The drawing under review shows one solid part. Ordinate dimensions are in mm from its lowest x, y, z. A direction names the side the tool comes from. Give positions to 0.01 mm unless a question says otherwise; leave off trailing zeros. Order: outer loops, then holes, each group sorted by start corner. A loop starts at its lowest first (then second) coordinate and runs counter-clockwise, first axis right, second up. Notation, with made-up numbers: (83.5, 15) -> (93.5, 15) arc R23 ccw to (93.5, 54) -> close; hole circle Ø9 at (75, 24.25). An arc over 180 degrees is marked (long way). One line per item, written item: value. Start each with the question number.
1) Consider section A-A (y = 16.5). State the section outline as (x, z) points.
2) Consider section D-D (y = 20). State the section outline as (x, z) points.
3) Consider section B-B (z = 8.25). State the section outline as (x, y) points.
4) Consider section C-C (x = 5). State the section outline as (y, z) points, plus the area to 3 significant figures.
5) Wall thickness on line 1 along Z through (x, y) = (7.75, 22.75); line 2 along Y through (x, z) = (5, 2.05); line 3 along X through (y, z) = (20, 3.9): over which ranges is each line inside the solid? List them lowest first. Write a range as from..to.
6) For pin 1 (0.9 mm diameter, centred on x = 5, z = 3.5, fed in from -Y); pin 2 (0.9 mm diameter, centred on x = 9, z = 8, fed in from +Y), all flat-tipped, find the tip position at first contact; note any pin that passes through.
7) Tool access review of the marked faces 1, 2 and 3: name each direction out of +Z, -Z, +X, -X, +Y, -Y from which nothing blocks a thin tool from reaching the whole face with its end or side.
8) The part is to be moulded in two halves that separate along Y. For the marked faces 4, 5 and 6, say which applies: released by +Y, released by -Y, zero draft, split by the parting line, or undercut.
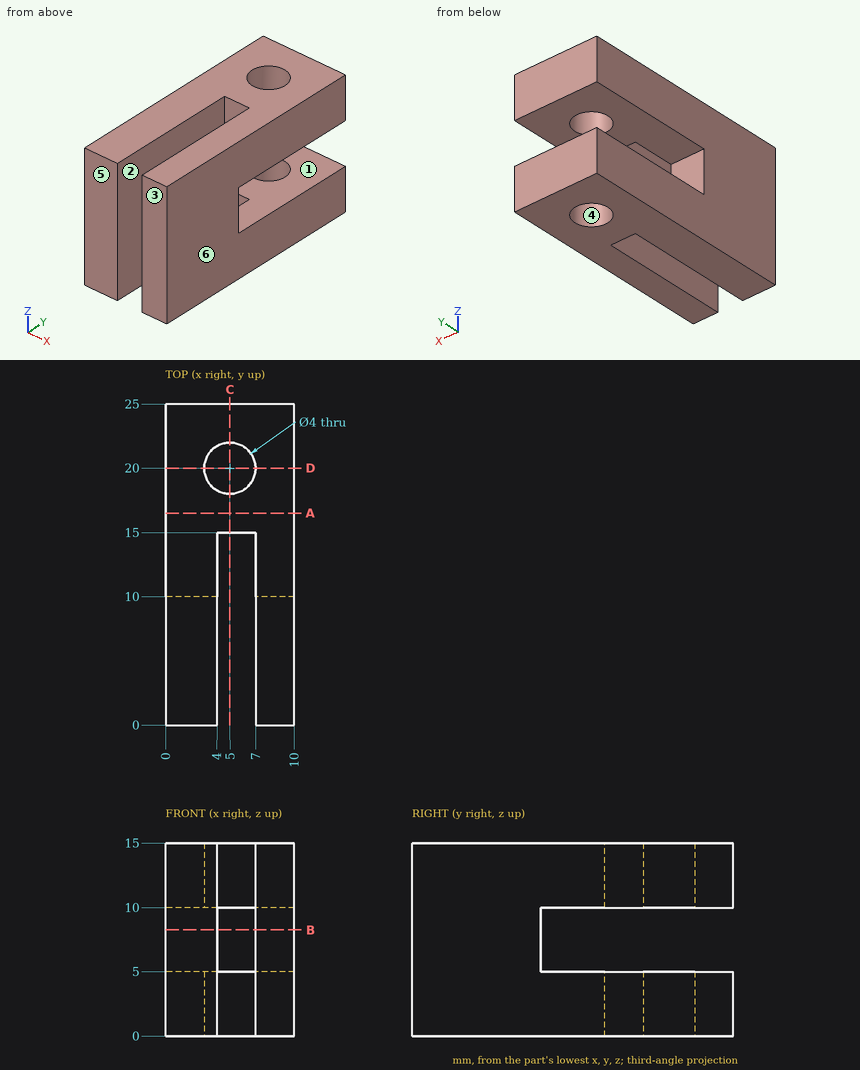
Checked values:
1. outline: (0, 0) -> (10, 0) -> (10, 5) -> (0, 5) -> close; (0, 10) -> (10, 10) -> (10, 15) -> (0, 15) -> close
2. outline: (0, 0) -> (3, 0) -> (3, 5) -> (0, 5) -> close; (0, 10) -> (3, 10) -> (3, 15) -> (0, 15) -> close; (7, 0) -> (10, 0) -> (10, 5) -> (7, 5) -> close; (7, 10) -> (10, 10) -> (10, 15) -> (7, 15) -> close
3. outline: (0, 0) -> (4, 0) -> (4, 10) -> (0, 10) -> close; (7, 0) -> (10, 0) -> (10, 10) -> (7, 10) -> close
4. outline: (15, 0) -> (18, 0) -> (18, 5) -> (15, 5) -> close; (15, 10) -> (18, 10) -> (18, 15) -> (15, 15) -> close; (22, 0) -> (25, 0) -> (25, 5) -> (22, 5) -> close; (22, 10) -> (25, 10) -> (25, 15) -> (22, 15) -> close
4. area: 60.0 mm^2
5. line 1: z = 0..5, 10..15
5. line 2: y = 15..18, 22..25
5. line 3: x = 0..3, 7..10
6. pin 1: stops at y = 15
6. pin 2: stops at y = 10
7. face 1: +X, -X, +Y
7. face 2: +Z, -Z, -Y
7. face 3: +Z, -Z, +X, -X, -Y
8. face 4: undercut
8. face 5: released by -Y
8. face 6: zero draft
